from build123d import *

# Parameters (mm, degrees)
F0_W      = 165.181708
F0_H      = 148.92931
F0_R      = 50.8
F1_DEPTH  = 3
F2_DEPTH  = 75
F1_FACE_W = 165.181708
F1_FACE_H = 148.92931
F3_DEPTH  = 7


with BuildPart() as f1:
    # F0 (on Front) → F1 (new body)
    with BuildSketch(Plane.XZ):
        Rectangle(F0_W, F0_H)
        Circle(F0_R, mode=Mode.SUBTRACT)
        Circle(F0_R)
    extrude(amount=F1_DEPTH)

    # F0 (on Front) → F2 (join)
    with BuildSketch(Plane.XZ):
        Circle(F0_R)
    extrude(amount=F2_DEPTH)

    # F1_face (on face) → F3 (join)
    with BuildSketch(Plane(origin=(0, 0, 0), x_dir=(1, 0, 0), z_dir=(0, 1, 0))):
        Rectangle(F1_FACE_W, F1_FACE_H)
    extrude(amount=F3_DEPTH)


solid = f1.part
Read the model definition and answer for the solid it produces. Units are mm, in the model's axes. A direction names the side the tool comes from. Give positions to 0.01 mm unless a question says otherwise; leave off trailing zeros. Write each loop counter-clockwise with the first axis right and the second up, starting at its lowest first coordinate (ties: lowest second). Pieces come first, ordered by that corner, then holes. Notation, with made-up numbers: (-21.5, 69) -> (-12.5, 69) arc R19 cw to (-12.5, 87) -> close; hole circle Ø10 at (89.5, 22.25). An arc over 180 degrees is marked (long way). Answer as a JSON object with one key per item and string values. Group by question number.
1) Consider L1, parallel to Y at x = -34, z = -55; L2, parallel to X at y = -51.5, z = 19; L3, parallel to X at y = -37, z = -6.5. Determine where each line is inside the solid, lowest interval first. Write a range as from..to.
2) A tool of negligible diameter and unlimited length cuts with its end or side. For faces 1 (the flat face through (-1, 2, 74.465)), 2 (the flat face through (-38, -3, 34)), from which of +Z, -Z, +X, -X, +Y, -Y can it reach the whole face along a straight path? Write none if from no direction.
3) Find section A-A (z = 0). Write down the section's boundary in (x, y).
4) Find section D-D (z = -61). Write down the section's boundary in (x, y), and give its area (3 significant figures).
5) Find section C-C (y = -44). Write down the section's boundary in (x, z).
6) Find section B-B (x = 0). Write down the section's boundary in (y, z).
7) Each of these flat-tipped pins is pushed along its axis until it touches: P1, Ø8, axis at y = -30, z = 50, coming from the +X side; P2, Ø3, axis at x = -34.5, y = -14, coming from the -Z side; P3, Ø1.5, axis at y = -51.5, z = 36, coming from the -X side. Where does it stop, or does it pass through?
Values follow:
{
 "1": {"L1": "y = -3..7", "L2": "x = -47.11..47.11", "L3": "x = -50.38..50.38"},
 "2": {"face 1": "+Z, +X, -X, +Y, -Y", "face 2": "-Y"},
 "3": {"outline": "(-82.59, -3) -> (-50.8, -3) -> (-50.8, -75) -> (50.8, -75) -> (50.8, -3) -> (82.59, -3) -> (82.59, 7) -> (-82.59, 7) -> close"},
 "4": {"outline": "(-82.59, -3) -> (82.59, -3) -> (82.59, 7) -> (-82.59, 7) -> close", "area": "1,650 mm2"},
 "5": {"outline": "circle Ø101.6 at (0, 0)"},
 "6": {"outline": "(-75, -50.8) -> (-3, -50.8) -> (-3, -74.46) -> (7, -74.46) -> (7, 74.46) -> (-3, 74.46) -> (-3, 50.8) -> (-75, 50.8) -> close"},
 "7": {"P1": "stops at x = 21.56", "P2": "stops at z = -38.62", "P3": "stops at x = -36.58"}
}
